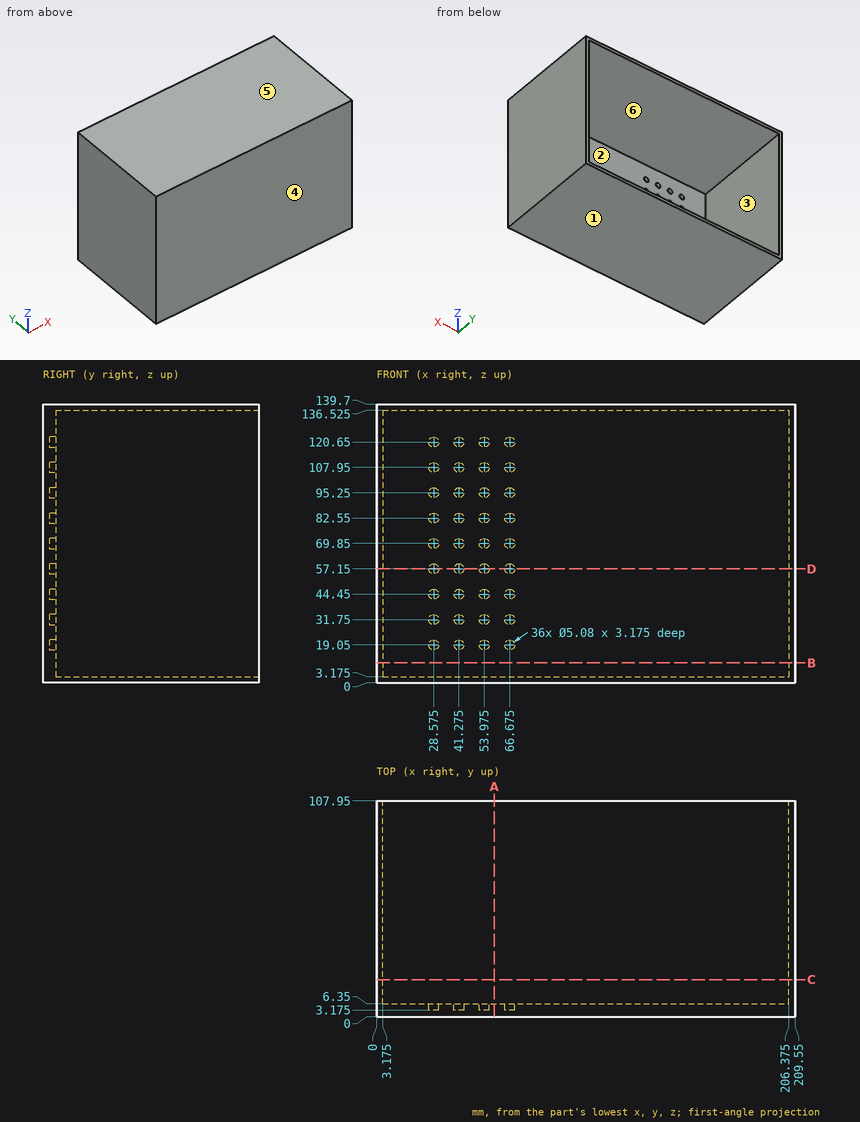
Study the drawing (mm; zero at the part's minimum x, y, z) and answer. A direction names the side the tool comes from. Round coordinates to 2 decimals unless told otherwise and drop trailing zeros. Loops run counter-clockwise (first coordinate to the right, second up) from the corner with the lowest first, then second, coordinate; pieces in that order, holes last. Notation, with made-up numbers: (71, 18) -> (98, 18) arc R27 cw to (98, 42) -> close; hole circle Ø5 at (24.5, 80.25). An arc over 180 degrees is marked (long way). One line per item, written item: value.
1) A cutting plane is placed at A-A (x = 59). Determine the outline of the cut face in (y, z) (3 decimals).
Answer list:
outline: (0, 0) -> (107.95, 0) -> (107.95, 3.175) -> (6.35, 3.175) -> (6.35, 136.525) -> (107.95, 136.525) -> (107.95, 139.7) -> (0, 139.7) -> close
2) A cutting plane is placed at B-B (z = 10). Determine the outline of the cut face in (x, y) (3 decimals), and give its area (3 significant figures).
Answer list:
outline: (0, 0) -> (209.55, 0) -> (209.55, 107.95) -> (206.375, 107.95) -> (206.375, 6.35) -> (3.175, 6.35) -> (3.175, 107.95) -> (0, 107.95) -> close
area: 1,980 mm²
3) For the marked faces 1 and 2, determine the directions among +Z, -Z, +X, -X, +Y, -Y from which every point of the face is accessible in a straight line to the end or side of a thin tool.
Answer list:
face 1: -Z, +X, -X, +Y, -Y
face 2: +Y
4) Flat-ended cylindrical pins translate along their axes: P1, Ø1.5, axis at x = 41.5, z = 57.5, coming from the +Y side (3 decimals); P2, Ø2, axis at x = 48.5, z = 97, coming from the +Y side. Find the tip coordinate at first contact, or state that the pin passes through.
Answer list:
P1: stops at y = 3.175
P2: stops at y = 6.35
5) Consider L1, parallel to X at y = 4.45, z = 95.25 (3 decimals); L2, parallel to X at y = 34, z = 20.5 (3 decimals); L3, parallel to Z at x = 164.5, y = 60.5 (3 decimals). Determine where each line is inside the solid, lowest interval first. Write a range as [from, to].
Answer list:
L1: x = [0, 26.035], [31.115, 38.735], [43.815, 51.435], [56.515, 64.135], [69.215, 209.55]
L2: x = [0, 3.175], [206.375, 209.55]
L3: z = [0, 3.175], [136.525, 139.7]
6) A cutting plane is placed at C-C (y = 18.5). Determine the outline of the cut face in (x, z) (3 decimals).
Answer list:
outline: (0, 0) -> (209.55, 0) -> (209.55, 139.7) -> (0, 139.7) -> close; hole (3.175, 3.175) -> (206.375, 3.175) -> (206.375, 136.525) -> (3.175, 136.525) -> close
7) A cutting plane is placed at D-D (z = 57.15). Determine the outline of the cut face in (x, y) (3 decimals), and give its area (3 significant figures).
Answer list:
outline: (0, 0) -> (209.55, 0) -> (209.55, 107.95) -> (206.375, 107.95) -> (206.375, 6.35) -> (69.215, 6.35) -> (69.215, 3.175) -> (64.135, 3.175) -> (64.135, 6.35) -> (56.515, 6.35) -> (56.515, 3.175) -> (51.435, 3.175) -> (51.435, 6.35) -> (43.815, 6.35) -> (43.815, 3.175) -> (38.735, 3.175) -> (38.735, 6.35) -> (31.115, 6.35) -> (31.115, 3.175) -> (26.035, 3.175) -> (26.035, 6.35) -> (3.175, 6.35) -> (3.175, 107.95) -> (0, 107.95) -> close
area: 1,910 mm²
8) The mould has two halves that part along Z. Classify the marked faces 3, 4, 5 and 6: pulls with the +Z half, pulls with the -Z half, needs draft (parallel to the pull), parting line crosses it, or undercut.
Answer list:
face 3: undercut
face 4: needs draft
face 5: pulls with the +Z half
face 6: undercut
